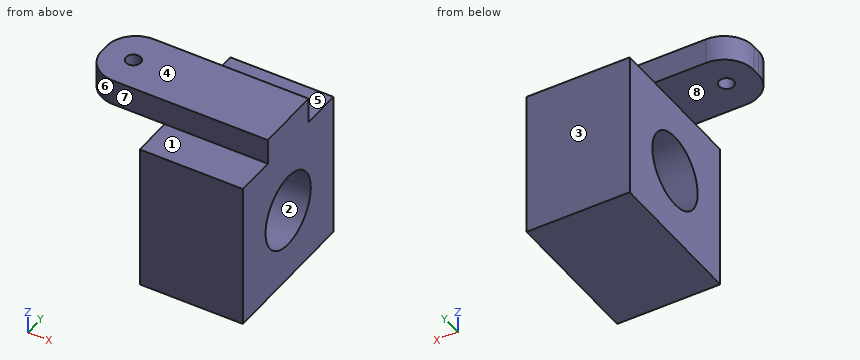
from build123d import *

# Parameters (mm, degrees)
AUFSATZ_LINEAR_AUSTRAGEN1_DEPTH      = 20
AUFSATZ_LINEAR_AUSTRAGEN1_DEPTH_BACK = 20
SKIZZE1_W                            = 28
SKIZZE1_H                            = 40
SKIZZE2_R                            = 10
SCHNITT_LINEAR_AUSTRAGEN1_DEPTH      = 40.799497484
SKIZZE3_W                            = 50
SKIZZE3_H                            = 18
AUFSATZ_LINEAR_AUSTRAGEN2_DEPTH      = 7
SKIZZE5_R                            = 2
SCHNITT_LINEAR_AUSTRAGEN2_DEPTH      = 63.4899992
VERRUNDUNG1_R                        = 8


with BuildPart() as part:
    # Skizze1 → Aufsatz-Linear austragen1 (new, two sides: drawn at the far end of the back side and taken through both)
    with BuildSketch(Plane(origin=(0, 0, 0), x_dir=(1, 0, 0), z_dir=(0, 1, 0)).offset(-AUFSATZ_LINEAR_AUSTRAGEN1_DEPTH_BACK)):
        Rectangle(SKIZZE1_W, SKIZZE1_H)
    extrude(amount=AUFSATZ_LINEAR_AUSTRAGEN1_DEPTH + AUFSATZ_LINEAR_AUSTRAGEN1_DEPTH_BACK)

    # Skizze2 → Schnitt-Linear austragen1 (cut, through all)
    with BuildSketch(Plane(origin=(14, 0, 0), x_dir=(0, 0, -1), z_dir=(1, 0, 0))):
        Circle(SKIZZE2_R)
    extrude(amount=-SCHNITT_LINEAR_AUSTRAGEN1_DEPTH, mode=Mode.SUBTRACT)

    # Skizze3 → Aufsatz-Linear austragen2 (add)
    with BuildSketch(Plane.XY.offset(20)):
        with Locations((-11, 0)):
            Rectangle(SKIZZE3_W, SKIZZE3_H)
    extrude(amount=AUFSATZ_LINEAR_AUSTRAGEN2_DEPTH)

    # Skizze5 → Schnitt-Linear austragen2 (cut, through all)
    with BuildSketch(Plane.XY.offset(27)):
        with Locations((-28, 0)):
            Circle(SKIZZE5_R)
    extrude(amount=-SCHNITT_LINEAR_AUSTRAGEN2_DEPTH, mode=Mode.SUBTRACT)

    # Verrundung1
    verrundung1_edges = [part.edges().sort_by_distance(p)[0] for p in [
        (-36, 9, 23.5),
        (-36, -9, 23.5),
    ]]
    fillet(verrundung1_edges, radius=VERRUNDUNG1_R)


solid = part.part
Read the model definition and answer for the solid it produces. Units are mm, in the model's axes. Face numbers are marked on the shaded views. A direction names the side the tool comes from. Coordinates: 2 decimals unless noted, no trailing zeros. Loops run counter-clockwise (first coordinate to the right, second up) from the corner with the lowest first, then second, coordinate; pieces in that order, holes last.
Q1. The part is cut by section A-A on y = 0. Write down the section's boundary in (x, z).
Q2. Each of these flat-tipped pins is pushed along its axis until it touches: pin 1 Ø2 at (x, z) = (3.5, 24) entering from +Y; pin 2 Ø12 at (x, y) = (-3.5, -15.5) entering from +Z; pin 3 Ø8 at (y, z) = (10, -5) entering from -X. Where does it stop, or does it pass through?
Q3. Which of the six approach directions +Z, -Z, +X, -X, +Y, -Y give full straight-line access (tool end or side, diameter ignored) to the marked faces 4, 5, 6, 7 and 8?
Q4. The part is cut by section B-B on z = 0. Write down the section's boundary in (x, y), and give its area (3 significant figures).
Q5. The part is cut by section D-D on z = 9. Write down the section's boundary in (x, y).
Q6. Consider probe 1 along Y at (x, z) = (-28, 21.5); probe 2 along Y at (x, z) = (4.5, 0); probe 3 along X at (y, z) = (13, 15). Determine where each line is inside the solid, lowest interval first.
Q7. The mould has two halves that part along Y. Classify the marked faces 1, 2 and 3: +Y half, -Y half, draft (parallel to the pull), parting line (faces both ways), or undercut.
Q8. The part is cut by section C-C on x = -1.5. Write down the section's boundary in (y, z), and give its area (3 significant figures).
Results below:
1. outline: (-36, 20) - (-30, 20) - (-30, 27) - (-36, 27) - close; (-26, 20) - (-14, 20) - (-14, 10) - (14, 10) - (14, 27) - (-26, 27) - close; (-14, -20) - (14, -20) - (14, -10) - (-14, -10) - close
2. pin 1: stops at y = 9
2. pin 2: stops at z = 20
2. pin 3: stops at x = -14
3. face 4: +Z, +X, -X, +Y, -Y
3. face 5: +Z, +X, -X, +Y
3. face 6: +Z, -Z, -X, -Y
3. face 7: +Z, +X, -X, -Y
3. face 8: -Z, -X, +Y, -Y
4. outline: (-14, -20) - (14, -20) - (14, -10) - (-14, -10) - close; (-14, 10) - (14, 10) - (14, 20) - (-14, 20) - close
4. area: 560 mm2
5. outline: (-14, -20) - (14, -20) - (14, -4.36) - (-14, -4.36) - close; (-14, 4.36) - (14, 4.36) - (14, 20) - (-14, 20) - close
6. probe 1: y = -9 to -2, 2 to 9
6. probe 2: y = -20 to -10, 10 to 20
6. probe 3: x = -14 to 14
7. face 1: draft
7. face 2: undercut
7. face 3: +Y half
8. outline: (-20, -20) - (20, -20) - (20, 20) - (9, 20) - (9, 27) - (-9, 27) - (-9, 20) - (-20, 20) - close; hole circle Ø20 at (0, 0)
8. area: 1,410 mm2
